```python
from build123d import *

# Parameters (mm, degrees)
EXTRUDE_1_DEPTH          = 50
CUT_EXTRUDE_1_DEPTH      = 27
CUT_EXTRUDE_1_DEPTH_BACK = 27
SKETCH_2_W               = 75
SKETCH_2_H               = 82


with BuildPart() as part:
    # Sketch 1 → Extrude 1 (new body)
    with BuildSketch(Plane.XY):
        Polygon((-27, 19.5), (-27, 10), (-26, 8.267949192), (-26, -14), (-15, -14), (-9, -20), (9, -20), (15, -14), (26, -14), (26, 8.267949192), (27, 10), (27, 19.5), (25.5, 21), (10.5, 21), (10, 20.5), (-10, 20.5), (-10.5, 21), (-25.5, 21), align=None)
    extrude(amount=EXTRUDE_1_DEPTH)

    # Sketch 2 → Cut-Extrude 1 (cut, two sides: drawn at the far end of the back side and taken through both)
    with BuildSketch(Plane(origin=(0, 0, 0), x_dir=(0, 0, -1), z_dir=(1, 0, 0)).offset(-CUT_EXTRUDE_1_DEPTH_BACK)):
        with Locations((-25, 0)):
            Rectangle(SKETCH_2_W, SKETCH_2_H)
        Polygon((-50, -20), (0, -20), (0, 20.5), (-0.5, 21), (-49.5, 21), (-50, 20.5), align=None, mode=Mode.SUBTRACT)
    extrude(amount=CUT_EXTRUDE_1_DEPTH + CUT_EXTRUDE_1_DEPTH_BACK, mode=Mode.SUBTRACT)

    # Sketch 3 → Cut-Revolve 1 (revolve, cut)
    with BuildSketch(Plane(origin=(0, 0, 0), x_dir=(0, 0, -1), z_dir=(1, 0, 0)), mode=Mode.PRIVATE) as cut_revolve_1_sk:
        Polygon((-50, 0), (-50, 16), (-47.2, 16), (-47.2, 16.85), (-45.85, 16.85), (-45.85, 16), (-4.15, 16), (-4.15, 16.85), (-2.8, 16.85), (-2.8, 16), (0, 16), (0, 0), align=None)
    revolve(cut_revolve_1_sk.sketch.rotate(Axis((0, 0, 0), (0, 0, 1)), 270), axis=Axis((0, 0, 0), (0, 0, 1)), mode=Mode.SUBTRACT)

    # Sketch 4 → Cut-Revolve 2 (revolve, cut)
    with BuildSketch(Plane(origin=(20, 0, 0), x_dir=(0, 0, -1), z_dir=(1, 0, 0)), mode=Mode.PRIVATE) as cut_revolve_2_sk:
        Polygon((-5, 21), (-2, 21), (-2.5415, 20.4585), (-2.5415, 9), (-2.4, 9), (-2.4, -13.5), (-2.111324865, -14), (-5, -14), align=None)
    revolve(cut_revolve_2_sk.sketch.rotate(Axis((20, -14, 5), (0, 1, 0)), 180), axis=Axis((20, -14, 5), (0, 1, 0)), mode=Mode.SUBTRACT)

    # Sketch 5 → Cut-Revolve 3 (revolve, cut)
    with BuildSketch(Plane(origin=(20, 0, 0), x_dir=(0, 0, -1), z_dir=(1, 0, 0)), mode=Mode.PRIVATE) as cut_revolve_3_sk:
        Polygon((-45, 21), (-42, 21), (-42.5415, 20.4585), (-42.5415, 9), (-42.4, 9), (-42.4, -13.5), (-42.111324865, -14), (-45, -14), align=None)
    revolve(cut_revolve_3_sk.sketch.rotate(Axis((20, -14, 45), (0, 1, 0)), 180), axis=Axis((20, -14, 45), (0, 1, 0)), mode=Mode.SUBTRACT)

    # Sketch 6 → Cut-Revolve 4 (revolve, cut)
    with BuildSketch(Plane(origin=(-20, 0, 0), x_dir=(0, 0, -1), z_dir=(1, 0, 0)), mode=Mode.PRIVATE) as cut_revolve_4_sk:
        Polygon((-5, 21), (-2, 21), (-2.5415, 20.4585), (-2.5415, 9), (-2.4, 9), (-2.4, -13.5), (-2.111324865, -14), (-5, -14), align=None)
    revolve(cut_revolve_4_sk.sketch.rotate(Axis((-20, -14, 5), (0, 1, 0)), 180), axis=Axis((-20, -14, 5), (0, 1, 0)), mode=Mode.SUBTRACT)

    # Sketch 7 → Cut-Revolve 5 (revolve, cut)
    with BuildSketch(Plane(origin=(-20, 0, 0), x_dir=(0, 0, -1), z_dir=(1, 0, 0)), mode=Mode.PRIVATE) as cut_revolve_5_sk:
        Polygon((-45, 21), (-42, 21), (-42.5415, 20.4585), (-42.5415, 9), (-42.4, 9), (-42.4, -13.5), (-42.111324865, -14), (-45, -14), align=None)
    revolve(cut_revolve_5_sk.sketch.rotate(Axis((-20, -14, 45), (0, 1, 0)), 180), axis=Axis((-20, -14, 45), (0, 1, 0)), mode=Mode.SUBTRACT)


solid = part.part
```
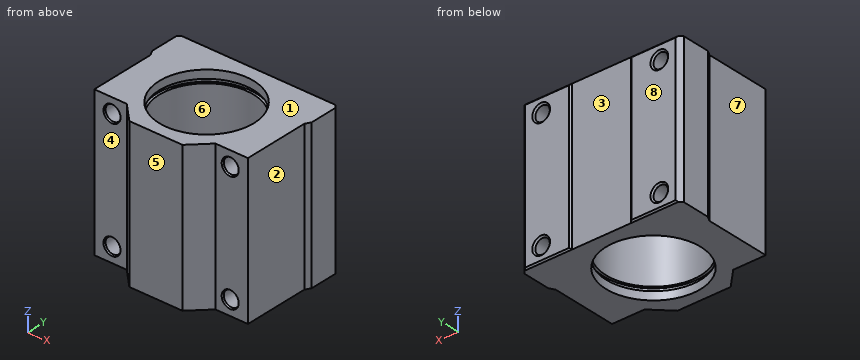
Here's how the part is built. I have some questions about the finished solid (model axes, mm). Face numbers are marked on the shaded views. A direction names the side the tool comes from. Round coordinates to 2 decimals unless told otherwise and drop trailing zeros. Order: outer loops, then holes, each group sorted by start corner. A loop starts at its lowest first (then second) coordinate and runs counter-clockwise, first axis right, second up. Notation, with made-up numbers: M -34,62 L -10,62 A20 cw -10,97 Z; hole C 74,17.5 d11. An arc over 180 degrees is marked long. Use CSV: the item, a comma, the result in double quotes.
1) I'm going to push flat-ended pins straight in: P1, Ø4, axis at y = 4.5, z = 14.5, coming from the +X side; P2, Ø5, axis at x = 0, z = 28, coming from the +Y side; P3, Ø7, axis at x = -20, z = 5, coming from the +Y side; P4, Ø18, axis at y = -0.5, z = 26, coming from the -X side. Where does each tip first touch, or does it pass through?
Taken from the geometry:
P1,"x = 26"
P2,"y = 20.5"
P3,"y = 21"
P4,"x = -26.13"
2) If we mould it in two halves opening along Y, with no side actions, what happens to the marked faces 5, 6, 7 and 8? For each: pulls with the +Y half, pulls with the -Y half, needs draft (parallel to the pull), parting line crosses it, or undercut.
Taken from the geometry:
face 5,"pulls with the -Y half"
face 6,"undercut"
face 7,"needs draft"
face 8,"pulls with the +Y half"
3) On a 3-axis mill with a long thin cutter (end or side, diameter ignored), from which of +Z, -Z, +X, -X, +Y, -Y can I reach the whole of each face in a straight line? I mean the marked faces 1, 2, 3 and 4. Say none if no direction works.
Taken from the geometry:
face 1,"+Z, +X, -X, +Y, -Y"
face 2,"+Z, -Z, +X, -Y"
face 3,"+Z, -Z, +Y"
face 4,"+Z, -Z, -X, -Y"
4) I want a section at D-D (z = 38). List the corners of the cut face in (x, y) for me, then the cut area to 3 significant figures.
Taken from the geometry:
outline,"M -27,10 L -26,8.27 L -26,-14 L -15,-14 L -9,-20 L 9,-20 L 15,-14 L 26,-14 L 26,8.27 L 27,10 L 27,19.5 L 25.5,21 L 10.5,21 L 10,20.5 L -10,20.5 L -10.5,21 L -25.5,21 L -27,19.5 Z; hole C 0,0 d32"
area,"1,170 mm^2"
5) I need wall thicknesses on line 1 along X through (y, z) = (12, 45); line 2 along X through (y, z) = (12.5, 44); line 3 along Y through (x, z) = (0, 46.75). Which ranges of each line are inside material? Lowest first, please. Write a range as [from, to].
Taken from the geometry:
line 1,"[-27, -22.46], [-17.54, -10.58], [10.58, 17.54], [22.46, 27]"
line 2,"[-27, -22.25], [-17.75, -9.99], [9.99, 17.75], [22.25, 27]"
line 3,"[-20, -16.85], [16.85, 20.5]"
6) I want a section at B-B (y = -7.5). List the corners of the cut face in (x, z) for me.
Taken from the geometry:
outline,"M -26,0 L -14.13,0 L -14.13,2.8 L -15.09,2.8 L -15.09,4.15 L -14.13,4.15 L -14.13,45.85 L -15.09,45.85 L -15.09,47.2 L -14.13,47.2 L -14.13,50 L -26,50 Z; M 14.13,0 L 26,0 L 26,50 L 14.13,50 L 14.13,47.2 L 15.09,47.2 L 15.09,45.85 L 14.13,45.85 L 14.13,4.15 L 15.09,4.15 L 15.09,2.8 L 14.13,2.8 Z; hole C -20,5 d5.2; hole C -20,45 d5.2; hole C 20,5 d5.2; hole C 20,45 d5.2"
7) I want a section at C-C (x = 20). Count the separate pieces of the cut face and the enclosed holes in it, then the cut area to 3 significant figures.
Taken from the geometry:
separate pieces,"3"
enclosed holes,"0"
area,"1,390 mm^2"
8) I want a section at A-A (x = 0). List the corners of the cut face in (y, z) for me.
Taken from the geometry:
outline,"M -20,0 L -16,0 L -16,2.8 L -16.85,2.8 L -16.85,4.15 L -16,4.15 L -16,45.85 L -16.85,45.85 L -16.85,47.2 L -16,47.2 L -16,50 L -20,50 Z; M 16,0 L 20.5,0 L 20.5,50 L 16,50 L 16,47.2 L 16.85,47.2 L 16.85,45.85 L 16,45.85 L 16,4.15 L 16.85,4.15 L 16.85,2.8 L 16,2.8 Z"
